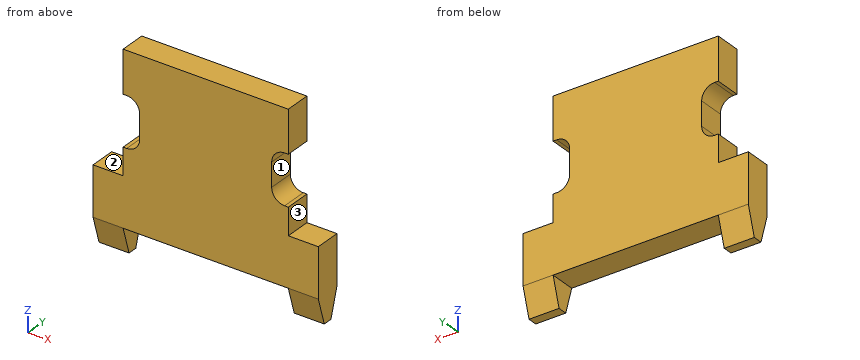
from build123d import *

# Parameters (mm, degrees)
F1_DEPTH  = 1.5875
F3_DEPTH  = 25.4
F4_W      = 1.5875
F4_H      = 3.048
F5_DEPTH  = 1.016
F6_R      = 0.79375
F7_W      = 1.5875
F7_H      = 3.048
F8_DEPTH  = 1.016
F9_R      = 0.79375
F10_DEPTH = 0.254


with BuildPart() as f1:
    # F0 (on Front) → F1 (new body)
    with BuildSketch(Plane.XZ):
        Polygon((-11.9713607894, 7.553705716), (-11.9713607894, 0), (-13.8092668185, 0), (-13.8092668185, -4.699), (-11.9713607894, -4.699), (-11.9713607894, -3.025394284), (-1.862878878, -3.025394284), (-1.862878878, -4.699), (-0.0249728489, -4.699), (-0.0249728489, 0), (-1.862878878, 0), (-1.862878878, 7.553705716), align=None)
    extrude(amount=F1_DEPTH)

    # F2 (on face) → F3 (cut)
    with BuildSketch(Plane(origin=(-13.8092668185, 0, 0), x_dir=(0, -1, 0), z_dir=(-1, 0, 0))):
        Polygon((0.508, -4.699), (0, -3.0226), (0, -4.699), align=None)
        Polygon((1.5875, -3.0226), (1.0795, -4.699), (1.5875, -4.699), align=None)
    extrude(amount=-F3_DEPTH, mode=Mode.SUBTRACT)

    # F4 (on face) → F5 (cut)
    with BuildSketch(Plane.YZ.offset(-1.862878878)):
        with Locations((-0.79375, 3.175)):
            Rectangle(F4_W, F4_H)
    extrude(amount=-F5_DEPTH, mode=Mode.SUBTRACT)

    # F6
    f6_edges = [f1.edges().sort_by_distance(p)[0] for p in [
        (-2.878879, -0.79375, 4.699),
        (-2.878879, -0.79375, 1.651),
    ]]
    fillet(f6_edges, radius=F6_R)

    # F7 (on face) → F8 (cut)
    with BuildSketch(Plane(origin=(-11.9713607894, 0, 0), x_dir=(0, -1, 0), z_dir=(-1, 0, 0))):
        with Locations((0.79375, 3.175)):
            Rectangle(F7_W, F7_H)
    extrude(amount=-F8_DEPTH, mode=Mode.SUBTRACT)

    # F9
    f9_edges = [f1.edges().sort_by_distance(p)[0] for p in [
        (-10.955361, -0.79375, 4.699),
        (-10.955361, -0.79375, 1.651),
    ]]
    fillet(f9_edges, radius=F9_R)

    # F10 (cut): a face of the model
    f10_faces = [f1.faces().sort_by_distance(p)[0] for p in [
        (-6.9171198337, -0.79375, 7.553705716),
    ]]
    extrude(f10_faces, amount=-F10_DEPTH, mode=Mode.SUBTRACT)


solid = f1.part
Verification items for the finished model (mm, model axes). Face numbers are marked on the shaded views. A direction names the side the tool comes from. Coordinates: 2 decimals unless noted, no trailing zeros. Loops run counter-clockwise (first coordinate to the right, second up) from the corner with the lowest first, then second, coordinate; pieces in that order, holes last. Notation, with made-up numbers: (34, 86.25) -> (75, 86.25) arc R33 cw to (75, 122.25) -> close; hole circle Ø8 at (-13, 41.5). An arc over 180 degrees is marked (long way). Answer as CSV lines item,"result".
1) Tool access check on the marked faces 1, 2 and 3. Record the directions out of +Z, -Z, +X, -X, +Y, -Y that give a thin tool (end or side, any length) a straight path to the whole face; none if there is none.
Found:
face 1,"+X, +Y, -Y"
face 2,"+Z, -X, +Y, -Y"
face 3,"+Z, +X, +Y, -Y"
2) Cross-section at B-B, the plane z = -3.25. Record the cut outline in (x, y), then the cut area to 3 significant figures.
Found:
outline,"(-13.81, -1.52) -> (-11.97, -1.52) -> (-11.97, -0.07) -> (-13.81, -0.07) -> close; (-1.86, -1.52) -> (-0.02, -1.52) -> (-0.02, -0.07) -> (-1.86, -0.07) -> close"
area,"5.33 mm2"
3) Cross-section at C-C, the plane y = -0.9. Record the cut outline in (x, z).
Found:
outline,"(-13.81, -4.7) -> (-11.97, -4.7) -> (-11.97, -3.03) -> (-1.86, -3.03) -> (-1.86, -4.7) -> (-0.02, -4.7) -> (-0.02, 0) -> (-1.86, 0) -> (-1.86, 1.65) -> (-2.09, 1.65) arc R0.79 cw to (-2.88, 2.44) -> (-2.88, 3.91) arc R0.79 cw to (-2.09, 4.7) -> (-1.86, 4.7) -> (-1.86, 7.3) -> (-11.97, 7.3) -> (-11.97, 4.7) -> (-11.75, 4.7) arc R0.79 cw to (-10.96, 3.91) -> (-10.96, 2.44) arc R0.79 cw to (-11.75, 1.65) -> (-11.97, 1.65) -> (-11.97, 0) -> (-13.81, 0) -> close"
4) Depth check by flat-ended pin: pin 1 (0.8 mm diameter, centred on y = -0.5, z = 1, fed in from +X); pin 2 (0.5 mm diameter, centred on y = -0.5, z = 6, fed in from -X); pin 3 (0.8 mm diameter, centred on x = -12.5, y = -0.5, fed in from +Z). Enter the tip coordinate at first touch or a pass-through.
Found:
pin 1,"stops at x = -1.86"
pin 2,"stops at x = -11.97"
pin 3,"stops at z = 0"
5) Thickness scan on L1, parallel to Z at x = -2, y = -0.1; L2, parallel to X at y = -0.75, z = 6.75; L3, parallel to Z at x = -3.25, y = -0.7. Record the ranges inside material, lowest first. Write a range as from..to.
Found:
L1,"z = -3.03..1.65, 4.7..7.3"
L2,"x = -11.97..-1.86"
L3,"z = -3.03..7.3"
